Can you work these out from the model? Positions are in its coordinate system, mm. A direction names the side the tool comes from. Round coordinates to 2 decimals unless told otherwise and drop trailing zeros. Write each loop counter-clockwise with the first axis right and the second up, starting at its lowest first coordinate (ties: lowest second). Pieces come first, ordered by that corner, then holes. Notation, with made-up numbers: (82.5, -30.5) -> (130.5, -30.5) arc R38 ccw to (130.5, 8.5) -> close; hole circle Ø9 at (-15, 6). An arc over 180 degrees is marked (long way). Write item = value, one per line. Start each with the question number.
1) I'm going to push flat-ended pins straight in: pin 1 (1.5 mm diameter, centred on y = -4, z = 2.5, fed in from -X); pin 2 (4 mm diameter, centred on x = -2, y = -1.5, fed in from -Z). Where does each tip first touch, or does it pass through?
2) Imagine slicing it at C-C, the plane z = 1.55. Please give me the cut outline in (x, y), then the cut area to 3 significant figures.
3) Imagine slicing it at D-D, the plane x = 6.5. Please give me the cut outline in (y, z).
4) If I drill on line 1 (Y direction, x = 0, z = 0.75); line 2 (Y direction, x = 0, z = 1.95); line 3 (Z direction, x = 5.25, y = 0.5), over which ranges is the centre line in solid material (lowest first)?
5) Imagine slicing it at B-B, the plane x = -2.5. Please give me the cut outline in (y, z).
6) Thinking about a two-plate mould opening in Y: for faces 3 (the face through (-1.73, -7.81, 1.48)), 4 (the face through (4, -6, 0)), 5 (the face through (6.466, -2.681, 0.493)), which applies, +Y half, -Y half, draft (parallel to the pull), parting line (faces both ways), or undercut?
7) Imagine slicing it at A-A, the plane y = 0. Please give me the cut outline in (x, z), then the cut area to 3 significant figures.
8) For faces 1 (the face through (0, -5, 1)), 2 (the face through (4.006, 1.262, 1.986)), which set-ups out of +Z, -Z, +X, -X, +Y, -Y let a thin tool reach every point of the face, with its end or its side?
from build123d import *

# Parameters (mm, degrees)
CYLINDER014005855_R     = 7
CYLINDER014005855_DEPTH = 1
TUBE004_R               = 8
TUBE004_R_2             = 4.2
TUBE004_DEPTH           = 3


with BuildPart() as obj1:
    # Cylinder014005855 → Cylinder014005855 (new body)
    with BuildSketch(Plane.XY):
        Circle(CYLINDER014005855_R)
    extrude(amount=CYLINDER014005855_DEPTH)


with BuildPart() as ring:
    # Tube004 → Tube004 (new body)
    with BuildSketch(Plane.XY):
        Circle(TUBE004_R)
        Circle(TUBE004_R_2, mode=Mode.SUBTRACT)
    extrude(amount=TUBE004_DEPTH)

    # Cut009003003007: cut obj1
    add(obj1.part, mode=Mode.SUBTRACT)


solid = ring.part
Reported:
q1.pin_1 = -7.31
q1.pin_2 = 1
q2.outline = circle Ø16 at (0, 0); hole circle Ø8.4 at (0, 0)
q2.area = 146 mm²
q3.outline = (-4.66, 0) -> (-2.6, 0) -> (-2.6, 1) -> (2.6, 1) -> (2.6, 0) -> (4.66, 0) -> (4.66, 3) -> (-4.66, 3) -> close
q4.line_1 = -8 to -7, 7 to 8
q4.line_2 = -8 to -4.2, 4.2 to 8
q4.line_3 = 1 to 3
q5.outline = (-7.6, 0) -> (-6.54, 0) -> (-6.54, 1) -> (-3.37, 1) -> (-3.37, 3) -> (-7.6, 3) -> close; (3.37, 1) -> (6.54, 1) -> (6.54, 0) -> (7.6, 0) -> (7.6, 3) -> (3.37, 3) -> close
q6.face_3 = parting line
q6.face_4 = draft
q6.face_5 = undercut
q7.outline = (-8, 0) -> (-7, 0) -> (-7, 1) -> (-4.2, 1) -> (-4.2, 3) -> (-8, 3) -> close; (4.2, 1) -> (7, 1) -> (7, 0) -> (8, 0) -> (8, 3) -> (4.2, 3) -> close
q7.area = 17.2 mm²
q8.face_1 = -Z
q8.face_2 = +Z, -Z
